Autodesk Inventor part; units mm, degrees
ref_plane "YZ Plane" through (0, 0, 0) normal (1, 0, 0) x (0, 1, 0)
ref_plane "XZ Plane" through (0, 0, 0) normal (0, 1, 0) x (-1, 0, 0)
ref_plane "XY Plane" through (0, 0, 0) normal (0, 0, 1) x (1, 0, 0)
sketch "Esboço1" plane through (0, 0, 0) normal (0, 0, 1) x (1, 0, 0)
  circle A0 centre (0, 0) radius 47.5
  circle A1 centre (0, 0) radius 57.5
  dimension "d0" = 95
  dimension "d1" = 115
extrude "Extrusão1" add sketch "Esboço1" against normal blind 15
sketch "Esboço2" plane through (0, 0, 0) normal (0, 0, 1) x (1, 0, 0)
  circle A0 centre (0, 8) radius 67.5
  circle A1 centre (0, 0) radius 47.5
  dimension "d4" = 135
  dimension "d5" = 8
extrude "Extrusão2" add sketch "Esboço2" along normal blind 20
sketch "Esboço3" plane through (0, 0, 0) normal (0, 1, 0) x (-1, 0, 0)
  line L0 (47.5, -15) -> (-47.5, -15)
  point P0 (0, 0)
  point P1 (0, -7)
  point P2 (0, -15)
  dimension "d8" = 8
hole "Furo1" at (0, 0, -7) direction (0, -1, 0) diameter 6.917 end through all
chamfer "Chanfro1" distance 0.5 angle 45 1 edges at (-0.0571, -57.5, -10.458)
pattern_circular "Padrão circular1" count 2 over 90 about axis through (0, 0, -10) along (0, 0, 1) of "Furo1"
chamfer "Chanfro2" distance 1.5 angle 45 1 edges at (-47.5, 0, -15)
chamfer "Chanfro3" distance 1 angle 45 5 edges at (-57.5, 0, -15) (-57.5, 0, 0) (-67.5, 8, 0) (-67.5, 8, 20) (-47.5, 0, 20)
Model file for the job. Use its own axes, mm. A direction names the side the tool comes from. Give positions to 0.01 mm unless a question says otherwise; leave off trailing zeros. Loops run counter-clockwise (first coordinate to the right, second up) from the corner with the lowest first, then second, coordinate; pieces in that order, holes last. Notation, with made-up numbers: (47, 4.25) -> (89, 4.25) arc R33 cw to (89, 39.25) -> close; hole circle Ø10 at (-19, -12.75). An arc over 180 degrees is marked (long way). Use a Markdown table: item, result. Add a question column.
(1) Tool access for faces 4 (the cylindrical face through (-12.465, -56.133, -7.409)), 5 (the cylindrical face through (52.51, -1.04, -3.7)), 6 (the cylindrical face through (-2.337, -52.254, -9.549)): list every direction of +Z, -Z, +X, -X, +Y, -Y with a clear straight run to the whole face (end or side of a thin tool).
(2) Mould opens along X. For faces 1 (the cylindrical face through (-53.57, 49.07, 9.87)), 2 (the flat face through (-15, 62, 0)), 3 (the cylindrical face through (-10.3, -46.37, 2.98)) say: +X half, -X half, draft (parallel to the pull), parting line (faces both ways), or undercut.
(3) Drop flat-ended pins along their axis: pin 1 Ø8 at (y, z) = (0, -7) entering from +X; pin 2 Ø1 at (x, z) = (-47.5, 0) entering from -Y; pin 3 Ø3 at (y, z) = (-6.5, 16) entering from -X. Give the stop position or say it passes through.
(4) Wall check: line 1 along Z through (x, y) = (0, -51); line 2 along Y through (x, z) = (0, 11.5); line 3 along Y through (x, z) = (-37, -5). Give the ranges that are in metal, low to high.
(5) Slice it at A-A on x = 0. Give the number of separate pieces and of enclosed holes in the cut face, and give its area (3 significant figures).
(6) Slice it at B-B on z = 17. List the corners of the cut face in (x, y), and give its area (3 significant figures).
Filled sheet:
| question | item | result |
|---|---|---|
| 1 | face 4 | -Z |
| 1 | face 5 | +X |
| 1 | face 6 | -Y |
| 2 | face 1 | parting line |
| 2 | face 2 | draft |
| 2 | face 3 | undercut |
| 3 | pin 1 | x = 57.5 |
| 3 | pin 2 | y = -39.41 |
| 3 | pin 3 | x = -66.24 |
| 4 | line 1 | -15 to -10.46, -3.54 to 20 |
| 4 | line 2 | -59.5 to -47.5, 47.5 to 75.5 |
| 4 | line 3 | -44.01 to -29.79, 29.79 to 44.01 |
| 5 | separate pieces | 3 |
| 5 | enclosed holes | 0 |
| 5 | area | 1,030 mm2 |
| 6 | outline | circle Ø135 at (0, 8); hole circle Ø95 at (0, 0) |
| 6 | area | 7,230 mm2 |
